Verification items for the finished model (mm, model axes). A direction names the side the tool comes from. Give positions to 0.01 mm unless a question says otherwise; leave off trailing zeros. Order: outer loops, then holes, each group sorted by start corner. A loop starts at its lowest first (then second) coordinate and runs counter-clockwise, first axis right, second up. Notation, with made-up numbers: (24, 60.25) -> (44, 60.25) arc R12 cw to (44, 72.25) -> close; hole circle Ø4 at (70.5, 7.5). An arc over 180 degrees is marked (long way). One line per question, with ' | ' between items. Start each with the question number.
Q1. Section check A-A on x = 0. Record the cut outline in (y, z).
Q2. Material ranges on probe 1 along Y at (x, z) = (-42.5, 95); probe 2 along Y at (x, z) = (-17, 13); probe 3 along Z at (x, y) = (14, -38.5), recorded low to high. Write a range as [from, to].
Q3. Section check B-B on y = -24.5. Record the cut outline in (x, z).
Q4. Section check C-C on z = 0. Record the cut outline in (x, y).
Q5. Go/stop test with flat-tipped pins: pin 1 (12 mm diameter, centred on y = -32.5, z = 18, fed in from -X); pin 2 (18 mm diameter, centred on x = 7.5, z = -12.5, fed in from +Y); pin 3 (1 mm diameter, centred on x = 65.5, z = -11, fed in from -Y). Record where each tip stops, or that it passes through.
Q6. Access from +Z, -Z, +X, -X, +Y, -Y to the whole of each face (thin tool, end or side, straight path). Record for faces 1 (the flat face through (0, -40.25, 0)), 2 (the conical face through (-37.667, -34.341, -4.946)), 3 (the flat face through (-1, -46.25, 1)), 4 (the cylindrical face through (-16.671, -43.232, 52.937)).
Q7. Mould release check, pull along Z, two halves, no side actions. Record for faces 5 (the flat face through (40, -6, -40)), 6 (the cylindrical face through (-130.2, -2.96, -141.99)), 7 (the conical face through (20.339, -29.351, -26.525)): released by +Z, released by -Z, zero draft, split by the parting line, or undercut.
Q8. Section check D-D on z = 127.5. Record the cut outline in (x, y).
from build123d import *


with BuildPart() as part:
    # Sketch1 → Revolve2 (revolve)
    with BuildSketch(Plane.XY, mode=Mode.PRIVATE) as revolve2_sk:
        Polygon((0, -40.25), (0, -46.25), (55.5, -46.25), (55.5, -40.29713119), (36.117911549, -40.29713119), (46.896841146, -6), (192.649801929, -6), (192.649801929, 0), (42.649801929, 0), (30, -40.25), align=None)
    revolve(revolve2_sk.sketch.rotate(Axis((0, -40.25, 0), (0, -1, 0)), 90), axis=Axis((0, -40.25, 0), (0, -1, 0)))


solid = part.part
Filled in:
1) outline: (-46.25, -55.5) -> (-40.3, -55.5) -> (-40.3, -36.12) -> (-6, -46.9) -> (-6, -192.65) -> (0, -192.65) -> (0, -42.65) -> (-40.25, -30) -> (-40.25, 30) -> (0, 42.65) -> (0, 192.65) -> (-6, 192.65) -> (-6, 46.9) -> (-40.3, 36.12) -> (-40.3, 55.5) -> (-46.25, 55.5) -> close
2) probe 1: [-6, 0] | probe 2: [-46.25, -40.25] | probe 3: [-33.91, -27.15], [27.15, 33.91]
3) outline: circle Ø82.17 at (0, 0); hole circle Ø69.9 at (0, 0)
4) outline: (-192.65, -6) -> (-46.9, -6) -> (-36.12, -40.3) -> (-55.5, -40.3) -> (-55.5, -46.25) -> (55.5, -46.25) -> (55.5, -40.3) -> (36.12, -40.3) -> (46.9, -6) -> (192.65, -6) -> (192.65, 0) -> (42.65, 0) -> (30, -40.25) -> (-30, -40.25) -> (-42.65, 0) -> (-192.65, 0) -> close
5) pin 1: x = -37.46 | pin 2: y = -40.25 | pin 3: y = -6
6) face 1: +Y | face 2: none | face 3: +Z, -Z, +X, -X, -Y | face 4: -Y
7) face 5: zero draft | face 6: split by the parting line | face 7: undercut
8) outline: (-144.42, -6) -> (144.42, -6) -> (144.42, 0) -> (-144.42, 0) -> close
